Geometry: final body of the model. Coordinates: model frame, mm. A direction names the side the tool comes from. Round coordinates to 2 decimals unless told otherwise and drop trailing zeros. Write each loop counter-clockwise with the first axis right and the second up, starting at its lowest first coordinate (ties: lowest second). Pieces come first, ordered by that corner, then holes. Notation, with made-up numbers: (49.25, -12) -> (108.25, -12) arc R12 cw to (108.25, 4) -> close; hole circle Ø6 at (15, 26.25). An arc over 180 degrees is marked (long way). One line per item, written item: value. Start each with the question number.
from build123d import *

# Parameters (mm, degrees)
SKETCH_1_R               = 17.02704374
EXTRUDE_1_DEPTH          = 6
SKETCH_1_6_R             = 17.02704374
EXTRUDE_2_DEPTH          = 8
SKETCH_1_7_R             = 19
EXTRUDE_3_DEPTH          = 1.5
CUT_EXTRUDE_START        = 1.5
CUT_EXTRUDE_3_DEPTH      = 27.535691538
PATTERN_CIRCULAR_1_COUNT = 22
HOLE_WIZARD_M4_1_D       = 4.3
PATTERN_CIRCULAR_2_COUNT = 6
HOLE_WIZARD_M5_1_D       = 5.3


with BuildPart() as part:
    # Sketch 1 → Extrude 1 (new body)
    with BuildSketch(Plane.XY):
        Circle(SKETCH_1_R)
    extrude(amount=EXTRUDE_1_DEPTH)

    # Sketch 1_6 → Extrude 2 (add)
    with BuildSketch(Plane.XY):
        Circle(SKETCH_1_6_R)
    extrude(amount=EXTRUDE_2_DEPTH)

    # Sketch 1_7 → Extrude 3 (add)
    with BuildSketch(Plane.XY):
        Circle(SKETCH_1_7_R)
    extrude(amount=EXTRUDE_3_DEPTH)

    # Sketch 3 → Cut-Extrude 3 (cut, through all)
    with BuildSketch(Plane.XY.offset(CUT_EXTRUDE_START)):
        with BuildLine():
            ThreePointArc((0.642707961, 15.103375051), (0, 15.11704374), (-0.642707961, 15.103375051))
            ThreePointArc((-0.642707961, 15.103375051), (-1.267879301, 15.950333421), (-1.58954065, 16.952686485))
            ThreePointArc((-1.58954065, 16.952686485), (0, 17.02704374), (1.58954065, 16.952686485))
            ThreePointArc((1.58954065, 16.952686485), (1.267879301, 15.950333421), (0.642707961, 15.103375051))
        make_face()
    cut_extrude_3 = extrude(amount=CUT_EXTRUDE_3_DEPTH, mode=Mode.SUBTRACT)

    # Pattern Circular 1: Cut-Extrude 3 ×22 about axis
    pattern_circular_1_axis = Axis((0, 0, 0), (0, 0, 1))
    for i in range(1, PATTERN_CIRCULAR_1_COUNT):
        add(cut_extrude_3.rotate(pattern_circular_1_axis, i * 360 / PATTERN_CIRCULAR_1_COUNT), mode=Mode.SUBTRACT)

    # Hole Wizard M4 _1 (through all)
    with Locations(Plane(origin=(0, 9, 8), x_dir=(1, 0, 0), z_dir=(0, 0, 1))):
        with Locations((0, 0)):
            hole_wizard_m4_1 = Hole(HOLE_WIZARD_M4_1_D / 2)

    # Pattern Circular 2: Hole Wizard M4 _1 ×6 about axis
    pattern_circular_2_axis = Axis((0, 0, 0), (0, 0, 1))
    for i in range(1, PATTERN_CIRCULAR_2_COUNT):
        add(hole_wizard_m4_1.rotate(pattern_circular_2_axis, i * 360 / PATTERN_CIRCULAR_2_COUNT), mode=Mode.SUBTRACT)

    # Hole Wizard M5 _1 (through all)
    with Locations(Plane(origin=(0, 0, 0), x_dir=(-1, 0, 0), z_dir=(0, 0, -1))):
        with Locations((0, 0)):
            Hole(HOLE_WIZARD_M5_1_D / 2)


solid = part.part
(1) Pin query (flat end, axial travel): pin 1 (8.5 mm diameter, centred on x = 0, y = 0, fed in from +Z); pin 2 (1.5 mm diameter, centred on x = -5, z = 3, fed in from +Y); pin 3 (1 mm diameter, centred on y = -5.5, z = 6, fed in from +X); pin 4 (1 mm diameter, centred on y = -8.5, z = 5, fed in from +X). Return the tip coordinate at first contact, or that it passes through.
(2) Line query: probe 1 along Y at (x, z) = (0, 3.25); probe 2 along Y at (x, z) = (-7, 0.75); probe 3 along X at (y, z) = (3, 4.5). Output: solid intervals per line, ascending.
(3) Section query A-A (x = 0). Output: boundary loops of the cut face in (y, z).
(4) Section query C-C (y = 4.5). Output: boundary loops of the cut face in (x, z).
(5) Section query B-B (y = 0). Output: boundary loops of the cut face in (x, z), and give its area (3 significant figures).
(6) Section query D-D (z = 6). Count the separate pieces of the cut face and the enclosed holes in it, and give its area (3 significant figures).
(7) Pull-direction query (X, two-part tool) for faces 4 (the face through (14, -7.8, 4.7)), 5 (the face through (-11.141, 12.876, 4.704)), 6 (the face through (-7.555, -14.089, 4.704)); classes: pulls with the +X half, pulls with the -X half, needs draft (parallel to the pull), parting line crosses it, or undercut.
(8) Set-up query: faces 1 (the face through (12.9, 9.49, 4.7)), 2 (the face through (-15.05, -5.472, 4.704)), 3 (the face through (4.25, -14.507, 4.704)). Return all of +Z, -Z, +X, -X, +Y, -Y with unobstructed straight access to the full face (end or side cutting, diameter ignored); none if empty.
Results list:
1. pin 1: stops at z = 8
1. pin 2: stops at y = 14.99
1. pin 3: stops at x = 16.28
1. pin 4: stops at x = 14.76
2. probe 1: y = -15.12 to -11.15, -6.85 to -2.65, 2.65 to 6.85, 11.15 to 15.12
2. probe 2: y = -17.66 to -6.5, -2.5 to 2.5, 6.5 to 17.66
2. probe 3: x = -15.03 to -9.33, -6.25 to 6.25, 9.33 to 15.03
3. outline: (-19, 0) -> (-11.15, 0) -> (-11.15, 8) -> (-15.12, 8) -> (-15.12, 1.5) -> (-19, 1.5) -> close; (-6.85, 0) -> (-2.65, 0) -> (-2.65, 8) -> (-6.85, 8) -> close; (2.65, 0) -> (6.85, 0) -> (6.85, 8) -> (2.65, 8) -> close; (11.15, 0) -> (19, 0) -> (19, 1.5) -> (15.12, 1.5) -> (15.12, 8) -> (11.15, 8) -> close
4. outline: (-18.46, 0) -> (-9.94, 0) -> (-9.94, 8) -> (-16.42, 8) -> (-16.42, 1.5) -> (-18.46, 1.5) -> close; (-5.64, 0) -> (5.64, 0) -> (5.64, 8) -> (-5.64, 8) -> close; (9.94, 0) -> (18.46, 0) -> (18.46, 1.5) -> (16.42, 1.5) -> (16.42, 8) -> (9.94, 8) -> close
5. outline: (-19, 0) -> (-2.65, 0) -> (-2.65, 8) -> (-17.03, 8) -> (-17.03, 1.5) -> (-19, 1.5) -> close; (2.65, 0) -> (19, 0) -> (19, 1.5) -> (17.03, 1.5) -> (17.03, 8) -> (2.65, 8) -> close
5. area: 236 mm^2
6. separate pieces: 1
6. enclosed holes: 7
6. area: 697 mm^2
7. face 4: pulls with the +X half
7. face 5: pulls with the -X half
7. face 6: undercut
8. face 1: +Z, +Y
8. face 2: +Z
8. face 3: +Z, -Y
